Geometry: final body of the model. Coordinates: model frame, mm. A direction names the side the tool comes from. Round coordinates to 2 decimals unless told otherwise and drop trailing zeros. Loops run counter-clockwise (first coordinate to the right, second up) from the corner with the lowest first, then second, coordinate; pieces in that order, holes last. Notation, with made-up numbers: M 73.25,2.5 L 125.25,2.5 A9 ccw 125.25,15.5 Z; hole C 50,46.25 d2. An arc over 180 degrees is marked long. Answer as a JSON object with one key per item and string values.
```python
from build123d import *

# Parameters (mm, degrees)
BOSS_EXTRUDE1_DEPTH = 16
FILLET1_R           = 8
FILLET2_R           = 10
SKETCH2_R           = 2.25
CUT_EXTRUDE1_DEPTH  = 13.7


with BuildPart() as part:
    # Sketch1 → Boss-Extrude1 (new body)
    with BuildSketch(Plane(origin=(0, 0, 0), x_dir=(1, 0, 0), z_dir=(0, 1, 0))):
        Polygon((0, 0), (211.9, 0), (211.9, 10.7), (213.9, 10.7), (213.9, -2), (-2, -2), (-2, 10.7), (0, 10.7), align=None)
    extrude(amount=BOSS_EXTRUDE1_DEPTH)

    # Fillet1
    fillet1_edges = [part.edges().sort_by_distance(p)[0] for p in [
        (0, 8, 0),
        (211.9, 8, 0),
    ]]
    fillet(fillet1_edges, radius=FILLET1_R)

    # Fillet2
    fillet2_edges = [part.edges().sort_by_distance(p)[0] for p in [
        (213.9, 8, 2),
        (-2, 8, 2),
    ]]
    fillet(fillet2_edges, radius=FILLET2_R)

    # Sketch2 → Cut-Extrude1 (cut, through all)
    with BuildSketch(Plane.XY.offset(2)):
        with Locations((17.95, 8)):
            Circle(SKETCH2_R)
        with Locations((193.95, 8)):
            Circle(SKETCH2_R)
    extrude(amount=-CUT_EXTRUDE1_DEPTH, mode=Mode.SUBTRACT)


solid = part.part
```
1) First-contact query: pin 1 (1 mm diameter, centred on y = 14, z = 0.5, fed in from +X); pin 2 (6 mm diameter, centred on x = 193.95, y = 8, fed in from -Z). Flat tips, straight axial feed; report the tip coordinate or a pass-through.
Geometry results:
{"pin 1": "x = 209.9", "pin 2": "z = 0"}
2) Pull-direction query (X, two-part tool) for faces 3 (the face through (211.05, 8.11, -1.01)), 4 (the face through (2.406, 8.112, -2.281)), 5 (the face through (106, 0, 1)); classes: +X half, -X half, draft (parallel to the pull), parting line (faces both ways), or undercut.
Geometry results:
{"face 3": "+X half", "face 4": "undercut", "face 5": "draft"}
3) Set-up query: faces 1 (the face through (209.494, 8.112, -2.281)), 2 (the face through (0.85, 8.11, -1.01)). Return all of +Z, -Z, +X, -X, +Y, -Y with unobstructed straight access to the full face (end or side cutting, diameter ignored); none if empty.
Geometry results:
{"face 1": "-Z, +Y, -Y", "face 2": "+Z, -X, +Y, -Y"}
4) Line query: probe 1 along Y at (x, z) = (17.95, 1.65); probe 2 along X at (y, z) = (10.5, -7.75); probe 3 along Z at (x, y) = (95.5, 1). Output: solid intervals per line, ascending.
Geometry results:
{"probe 1": "0 to 5.75, 10.25 to 16", "probe 2": "-2 to 0, 211.9 to 213.9", "probe 3": "0 to 2"}
5) Cut plane B-B on x = 17.95. Return the cut outline in (y, z), and give its area (3 significant figures).
Geometry results:
{"outline": "M 0,0 L 5.75,0 L 5.75,2 L 0,2 Z; M 10.25,0 L 16,0 L 16,2 L 10.25,2 Z", "area": "23.0 mm2"}
6) Cut plane A-A on y = 8. Return the cut outline in (x, z).
Geometry results:
{"outline": "M -2,-10.7 L 0,-10.7 L 0,-8 A8 cw 8,0 L 15.7,0 L 15.7,2 L 8,2 A10 ccw -2,-8 Z; M 20.2,0 L 191.7,0 L 191.7,2 L 20.2,2 Z; M 196.2,0 L 203.9,0 A8 cw 211.9,-8 L 211.9,-10.7 L 213.9,-10.7 L 213.9,-8 A10 ccw 203.9,2 L 196.2,2 Z"}
7) Cut plane C-C on x = 109.5. Return the cut outline in (y, z), and give its area (3 significant figures).
Geometry results:
{"outline": "M 0,0 L 16,0 L 16,2 L 0,2 Z", "area": "32.0 mm2"}
